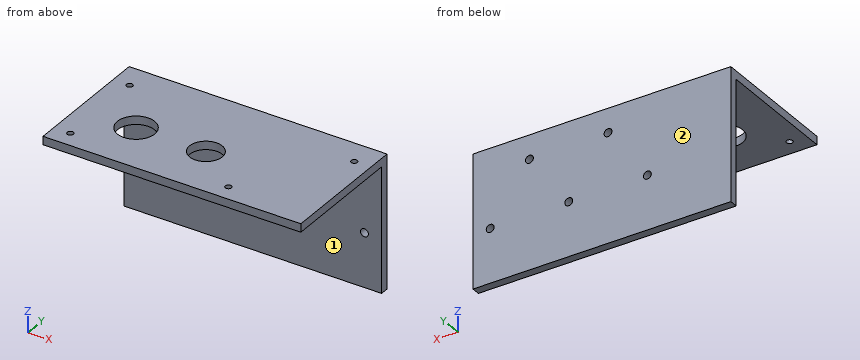
```python
from build123d import *

# Parameters (mm, degrees)
SKETCH1_W           = 196.85
SKETCH1_H           = 101.6
SKETCH1_R           = 2.999999969
BOSS_EXTRUDE1_DEPTH = 6.35
SKETCH2_W           = 196.85
SKETCH2_H           = 6.35
BOSS_EXTRUDE2_DEPTH = 95.25
SKETCH4_R           = 12.500000019
SKETCH4_R_2         = 2.38125
SKETCH4_R_3         = 14.2875
CUT_EXTRUDE1_DEPTH  = 183.917715111


with BuildPart() as part:
    # Sketch1 → Boss-Extrude1 (new body)
    with BuildSketch(Plane(origin=(0, 0, 0), x_dir=(1, 0, 0), z_dir=(0, 1, 0))):
        with Locations((-25.3238, -1.549999948)):
            Rectangle(SKETCH1_W, SKETCH1_H)
        with Locations(Location((-59.999999888, 8.000000002, 0), (0, 0, 270))):
            Circle(SKETCH1_R, mode=Mode.SUBTRACT)
        with Locations(Location((0, 8.000000002, 0), (0, 0, 270))):
            Circle(SKETCH1_R, mode=Mode.SUBTRACT)
        with Locations(Location((59.999999888, 8.000000002, 0), (0, 0, 270))):
            Circle(SKETCH1_R, mode=Mode.SUBTRACT)
        with Locations(Location((29.999999944, -34.000000072, 0), (0, 0, 270))):
            Circle(SKETCH1_R, mode=Mode.SUBTRACT)
        with Locations(Location((-29.999999944, -34.000000072, 0), (0, 0, 270))):
            Circle(SKETCH1_R, mode=Mode.SUBTRACT)
    extrude(amount=BOSS_EXTRUDE1_DEPTH)

    # Sketch2 → Boss-Extrude2 (add)
    with BuildSketch(Plane.XZ):
        with Locations((-25.3238, 49.174999948)):
            Rectangle(SKETCH2_W, SKETCH2_H)
    extrude(amount=BOSS_EXTRUDE2_DEPTH)

    # Sketch4 → Cut-Extrude1 (cut, through all)
    with BuildSketch(Plane(origin=(0, 0, 45.999999948), x_dir=(-1, 0, 0), z_dir=(0, 0, -1))):
        with Locations((26.098799974, -53.99999995)):
            Circle(SKETCH4_R)
        with Locations((-60.4012, -12.7)):
            Circle(SKETCH4_R_2)
        with Locations((111.0488, -12.7)):
            Circle(SKETCH4_R_2)
        with Locations((111.0488, -82.55)):
            Circle(SKETCH4_R_2)
        with Locations((-9.6012, -82.55)):
            Circle(SKETCH4_R_2)
        with Locations((79.438799974, -53.99999995)):
            Circle(SKETCH4_R_3)
    extrude(amount=-CUT_EXTRUDE1_DEPTH, mode=Mode.SUBTRACT)


solid = part.part
```
Verification items for the finished model (mm, model axes). Face numbers are marked on the shaded views. A direction names the side the tool comes from. Give positions to 0.01 mm unless a question says otherwise; leave off trailing zeros. Order: outer loops, then holes, each group sorted by start corner. A loop starts at its lowest first (then second) coordinate and runs counter-clockwise, first axis right, second up. Notation, with made-up numbers: (41, -1) - (82, -1) arc R28 ccw to (82, 27) - close; hole circle Ø10 at (8, 34). An arc over 180 degrees is marked (long way). Answer as CSV lines item,"result". Start each with the question number.
Item 1: Material ranges on L1, parallel to X at y = 2, z = -8; L2, parallel to X at y = 2, z = 34; L3, parallel to Y at x = -83.5, z = -18, recorded low to high.
Item 2: Section check A-A, the plane x = -60. Record the boundary of the cut face in (y, z), plus the area to 3 significant figures.
Item 3: Gauge pin test, flat ends, axial feed: pin 1 (3 mm diameter, centred on x = 53, z = 12.5, fed in from -Y); pin 2 (6 mm diameter, centred on x = 60.4, y = -12.7, fed in from -Z). Record the tip position at first contact, or that the pin passes through.
Item 4: Access from +Z, -Z, +X, -X, +Y, -Y to the whole of each face (thin tool, end or side, straight path). Record for the marked faces 1 and 2.
Item 5: Section check D-D, the plane x = -30. Record the boundary of the cut face in (y, z).
Item 6: Section check B-B, the plane z = -8. Record the boundary of the cut face in (x, y), plus the area to 3 significant figures.
Item 7: Section check C-C, the plane y = -82.55. Record the boundary of the cut face in (x, z).
Filled in:
1,L1,"-123.75 to -63, -57 to -3, 3 to 57, 63 to 73.1"
1,L2,"-123.75 to -33, -27 to 27, 33 to 73.1"
1,L3,"0 to 6.35"
2,outline,"(-95.25, 46) - (0, 46) - (0, -5) - (6.35, -5) - (6.35, 52.35) - (-95.25, 52.35) - close; (0, -49.25) - (6.35, -49.25) - (6.35, -11) - (0, -11) - close"
2,area,"1,210 mm^2"
3,pin 1,"y = 0"
3,pin 2,"z = 46"
4,face 1,"-Z, +X, -X, -Y"
4,face 2,"+Z, -Z, +X, -X, +Y"
5,outline,"(-95.25, 46) - (-65.88, 46) - (-65.88, 52.35) - (-95.25, 52.35) - close; (-42.12, 46) - (0, 46) - (0, 37) - (6.35, 37) - (6.35, 52.35) - (-42.12, 52.35) - close; (0, -49.25) - (6.35, -49.25) - (6.35, 31) - (0, 31) - close"
6,outline,"(-123.75, 0) - (-63, 0) - (-63, 6.35) - (-123.75, 6.35) - close; (-57, 0) - (-3, 0) - (-3, 6.35) - (-57, 6.35) - close; (3, 0) - (57, 0) - (57, 6.35) - (3, 6.35) - close; (63, 0) - (73.1, 0) - (73.1, 6.35) - (63, 6.35) - close"
6,area,"1,140 mm^2"
7,outline,"(-123.75, 46) - (-113.43, 46) - (-113.43, 52.35) - (-123.75, 52.35) - close; (-108.67, 46) - (7.22, 46) - (7.22, 52.35) - (-108.67, 52.35) - close; (11.98, 46) - (73.1, 46) - (73.1, 52.35) - (11.98, 52.35) - close"
